Could you check a few things on this model? Use its own coordinates, in mm. Face numbers are marked on the shaded views. A direction names the side the tool comes from. Round coordinates to 2 decimals unless told otherwise and drop trailing zeros. Loops run counter-clockwise (first coordinate to the right, second up) from the corner with the lowest first, then second, coordinate; pieces in that order, holes last. Notation, with made-up numbers: (-9, 28) -> (-4, 28) arc R23 ccw to (-4, 55) -> close; hole circle Ø7 at (61.5, 32.25). An arc over 180 degrees is marked (long way). One line per item, written item: value.
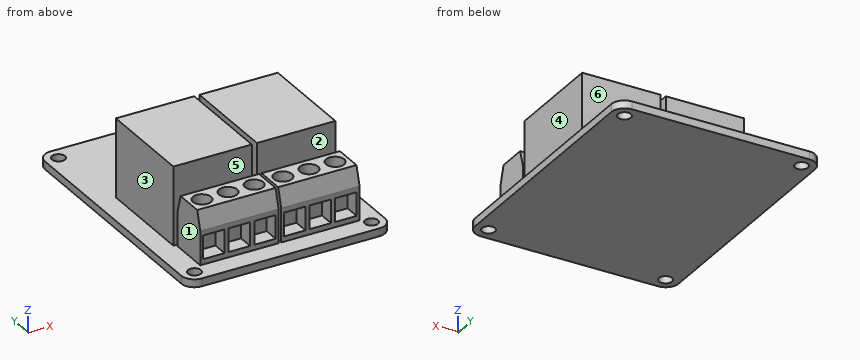
Autodesk Inventor part; units mm, degrees
ref_plane "YZ Plane" through (0, 0, 0) normal (1, 0, 0) x (0, 1, 0)
ref_plane "XZ Plane" through (0, 0, 0) normal (0, 1, 0) x (-1, 0, 0)
ref_plane "XY Plane" through (0, 0, 0) normal (0, 0, 1) x (1, 0, 0)
sketch "Sketch1" plane through (0, 0, 0) normal (0, 0, 1) x (1, 0, 0)
  line L0 (-17, -25) -> (17, -25)
  line L1 (19.5, -22.5) -> (19.5, 22.5)
  line L2 (17, 25) -> (-17, 25)
  line L3 (-19.5, 22.5) -> (-19.5, -22.5)
  line L4 (19.5, -25) -> (-19.5, 25) construction
  circle A0 centre (16.95, -22.45) radius 1.25
  arc A1 (17, -25) -> (19.5, -22.5) centre (17, -22.5) ccw
  circle A2 centre (-16.95, -22.45) radius 1.25
  circle A3 centre (-16.95, 22.45) radius 1.25
  circle A4 centre (16.95, 22.45) radius 1.25
  arc A5 (19.5, 22.5) -> (17, 25) centre (17, 22.5) ccw
  arc A6 (-17, 25) -> (-19.5, 22.5) centre (-17, 22.5) ccw
  arc A7 (-19.5, -22.5) -> (-17, -25) centre (-17, -22.5) ccw
  point P0 (0, 0)
  point P1 (-19.5, -25)
  point P2 (19.5, 25)
  point P3 (0, 0)
  dimension "d0" = 50
  dimension "d1" = 39
  dimension "d2" = 2.5
  dimension "d3" = 2.55
  dimension "d4" = 2.55
  dimension "d5" = 2.5
  dimension "d6" = 2.5
  dimension "d7" = 2.5
  dimension "d8" = 2.5
  dimension "d9" = 2.55
  dimension "d10" = 2.55
  dimension "d11" = 2.55
  dimension "d12" = 2.55
  dimension "d13" = 2.55
  dimension "d14" = 2.55
  dimension "d15" = 2.5
extrude "Extrusion1" add sketch "Sketch1" along normal blind 1.5
sketch "Sketch2" plane through (0, 0, 1.5) normal (0, 0, 1) x (1, 0, 0)
  line L0 (0.5, -13) -> (15.5, -13)
  line L1 (15.5, -13) -> (15.5, 6)
  line L2 (15.5, 6) -> (0.5, 6)
  line L3 (0.5, 6) -> (0.5, -13)
  line L4 (-15.5, -13) -> (-0.5, -13)
  line L5 (-0.5, -13) -> (-0.5, 6)
  line L6 (-0.5, 6) -> (-15.5, 6)
  line L7 (-15.5, 6) -> (-15.5, -13)
  line L8 (19.5, -22.5) -> (19.5, 22.5)
  line L9 (-19.5, 22.5) -> (-19.5, -22.5)
  line L10 (-17, -25) -> (17, -25)
  point P0 (0, 0)
  dimension "d18" = 15
  dimension "d19" = 19
  dimension "d22" = 16
  dimension "d27" = 4
  dimension "d28" = 39
  dimension "d29" = 12
extrude "Extrusion2" add sketch "Sketch2" along normal blind 15
sketch "Sketch3" plane through (0, 0, 1.5) normal (0, 0, 1) x (1, 0, 0)
  line L0 (0, -21) -> (-15, -21)
  line L1 (-15, -21) -> (-15, -13.5)
  line L2 (-15, -13.5) -> (0, -13.5)
  line L3 (0, -13.5) -> (0, -21)
  line L4 (-15.5, -13) -> (-0.5, -13)
  line L5 (-15.5, 6) -> (-15.5, -13)
  line L6 (15.5, -21) -> (0.5, -21)
  line L7 (0.5, -21) -> (0.5, -13.5)
  line L8 (0.5, -13.5) -> (15.5, -13.5)
  line L9 (15.5, -13.5) -> (15.5, -21)
  line L10 (0.5, -13) -> (15.5, -13)
  point P0 (0, 0)
  dimension "d32" = 15
  dimension "d33" = 7.5
  dimension "d34" = 0.5
  dimension "d35" = 0.5
  dimension "d36" = 15
  dimension "d37" = 7.5
  dimension "d38" = 0.5
  dimension "d39" = 0.5
extrude "Extrusion3" add sketch "Sketch3" along normal blind 10
chamfer "Chamfer1" distance 1 distance2 3.5 1 edges at (8, -21, 11.5) measured on face at (10.5, -18.5, 11.5)
chamfer "Chamfer2" distance 1 distance2 3.5 1 edges at (8, -13.5, 11.5) measured on face at (10.5, -17.8333, 11.5)
chamfer "Chamfer3" distance 1 distance2 3.5 1 edges at (-7.5, -13.5, 11.5) measured on face at (-5, -18.5, 11.5)
chamfer "Chamfer4" distance 1 distance2 3.5 1 edges at (-7.5, -21, 11.5) measured on face at (-5, -18.8333, 11.5)
sketch "Sketch4" plane through (0, 0, 11.5) normal (0, 0, 1) x (1, 0, 0)
  line L0 (0.5, -14.5) -> (0.5, -20)
  line L1 (0, -20) -> (0, -14.5)
  line L2 (0.25, -35.642) -> (0.25, -29.5385) construction
  circle A0 centre (-12.5, -17.25) radius 1.75
  line L3 (-15, -14.5) -> (-15, -20)
  line L4 (-15, -14.5) -> (0, -14.5)
  line L5 (0, -20) -> (-15, -20)
  circle A1 centre (-7.5, -17.25) radius 1.75
  circle A2 centre (-2.5, -17.25) radius 1.75
  circle A3 centre (13, -17.25) radius 1.75
  circle A4 centre (8, -17.25) radius 1.75
  circle A5 centre (3, -17.25) radius 1.75
  point P0 (0, 0)
  dimension "d54" = 0.5
  dimension "d55" = 0.25
  dimension "d56" = 3.5
  dimension "d57" = 2.5
  dimension "d58" = 5.5
  dimension "d59" = 2.75
  dimension "d62" = 5
extrude "Extrusion4" cut sketch "Sketch4" against normal blind 3 contours A0 | A1 | A2 | A3 | A4 | A5
sketch "Sketch5" plane through (0.5, -21, 1.5) normal (0, -1, 0) x (1, 0, 0)
  line L0 (0.55, 5.5) -> (4.65, 5.5)
  line L1 (4.65, 5.5) -> (4.65, 1)
  line L2 (4.65, 1) -> (0.55, 1)
  line L3 (0.55, 1) -> (0.55, 5.5)
  line L4 (15, 10) -> (0, 10)
  line L5 (0, 0) -> (0, 6.5)
  line L6 (5.45, 1) -> (5.45, 5.5)
  line L7 (5.45, 5.5) -> (9.55, 5.5)
  line L8 (9.55, 1) -> (5.45, 1)
  line L9 (9.55, 5.5) -> (9.55, 1)
  line L10 (10.35, 1) -> (10.35, 5.5)
  line L11 (10.35, 5.5) -> (14.45, 5.5)
  line L12 (14.45, 1) -> (10.35, 1)
  line L13 (14.45, 5.5) -> (14.45, 1)
  line L14 (15, 0) -> (15, 6.5)
  line L15 (-0.5, 0) -> (-0.5, 6.5)
  line L16 (-0.25, -5.4551) -> (-0.25, -7.5555) construction
  line L17 (-1.05, 5.5) -> (-5.15, 5.5)
  line L18 (-5.15, 5.5) -> (-5.15, 1)
  line L19 (-5.15, 1) -> (-1.05, 1)
  line L20 (-1.05, 1) -> (-1.05, 5.5)
  line L21 (-5.95, 1) -> (-5.95, 5.5)
  line L22 (-5.95, 5.5) -> (-10.05, 5.5)
  line L23 (-10.05, 1) -> (-5.95, 1)
  line L24 (-10.05, 5.5) -> (-10.05, 1)
  line L25 (-10.85, 1) -> (-10.85, 5.5)
  line L26 (-10.85, 5.5) -> (-14.95, 5.5)
  line L27 (-14.95, 1) -> (-10.85, 1)
  line L28 (-14.95, 5.5) -> (-14.95, 1)
  point P0 (-0.5, -1.5)
  dimension "d71" = 4.1
  dimension "d72" = 4.5
  dimension "d73" = 4.5
  dimension "d74" = 0.55
  dimension "d77" = 4.9
  dimension "d85" = 0.5
  dimension "d86" = 0.25
extrude "Extrusion5" cut sketch "Sketch5" against normal blind 3
equation "\"d4\" = d3"
equation "\"d5\" = d2"
equation "\"d6\" = d2"
equation "\"d7\" = d2"
equation "\"d8\" = d2"
equation "\"d9\" = d3"
equation "\"d10\" = d3"
equation "\"d11\" = d3"
equation "\"d12\" = d3"
equation "\"d13\" = d3"
equation "\"d14\" = d3"
equation "\"d15\" = d2"
equation "\"d27\" = -0.5 * d22 + 0.5 * d28 - 0.5 * d18"
equation "\"d39\" = d34"
equation "\"d55\" = 0.5 * d54"
equation "\"d59\" = 0.5 * d58"
equation "\"d86\" = 0.5 * d85"
properties part number "Dual Relay w Breakout Board"
(1) Please list where these lines run through material, in increasing order: L1, parallel to Y at x = 16.95, z = 1.2; L2, parallel to X at y = -6, z = 2.5; L3, parallel to Y at x = 8, z = 10.7.
Results below:
L1: y = -25 to -23.7, -21.2 to 21.2, 23.7 to 25
L2: x = -15.5 to -0.5, 0.5 to 15.5
L3: y = -20.23 to -19, -15.5 to -14.27, -13 to 6
(2) Imagine slicing it at C-C on y = -3. Write out the boundary of the cut face in (x, z).
Results below:
outline: (-19.5, 0) -> (19.5, 0) -> (19.5, 1.5) -> (15.5, 1.5) -> (15.5, 16.5) -> (0.5, 16.5) -> (0.5, 1.5) -> (-0.5, 1.5) -> (-0.5, 16.5) -> (-15.5, 16.5) -> (-15.5, 1.5) -> (-19.5, 1.5) -> close
(3) Imagine slicing it at B-B on x = 3. Write out the boundary of the cut face in (y, z).
Results below:
outline: (-25, 0) -> (25, 0) -> (25, 1.5) -> (6, 1.5) -> (6, 16.5) -> (-13, 16.5) -> (-13, 1.5) -> (-13.5, 1.5) -> (-13.5, 8) -> (-14.5, 11.5) -> (-15.5, 11.5) -> (-15.5, 8.5) -> (-19, 8.5) -> (-19, 11.5) -> (-20, 11.5) -> (-21, 8) -> (-21, 7) -> (-18, 7) -> (-18, 2.5) -> (-21, 2.5) -> (-21, 1.5) -> (-25, 1.5) -> close
(4) Imagine slicing it at D-D on z = 3.75. Give the number of separate pieces and of enclosed holes in the cut face, then the cut area to 3 significant figures.
Results below:
separate pieces: 4
enclosed holes: 0
area: 721 mm²
(5) Imagine slicing it at A-A on z = 12.5. Write out the boundary of the cut face in (x, y), then the cut area to 3 significant figures.
Results below:
outline: (-15.5, -13) -> (-0.5, -13) -> (-0.5, 6) -> (-15.5, 6) -> close; (0.5, -13) -> (15.5, -13) -> (15.5, 6) -> (0.5, 6) -> close
area: 570 mm²
(6) On a 3-axis mill with a long thin cutter (end or side, diameter ignored), from which of +Z, -Z, +X, -X, +Y, -Y can I reach the whole of each face in a straight line? I mean the marked faces 1, 2 and 3. Say none if no direction works.
Results below:
face 1: +Z, -X, -Y
face 2: +Z, +X, -X
face 3: +Z, -X, +Y, -Y
(7) For pin 1 Ø4 at (x, z) = (5.5, 11) entering from -Y; pin 2 Ø2 at (x, z) = (13.5, 5.5) entering from -Y; pin 3 Ø6 at (x, y) = (7, -16.5) entering from +Z; pin 4 Ø1.5 at (x, y) = (2.5, -19) entering from -Z, each with a flat end and sliding along its axis, tell me the tip position at first contact or that it passes through.
Results below:
pin 1: stops at y = -20.71
pin 2: stops at y = -18
pin 3: stops at z = 11.5
pin 4: stops at z = 0
(8) We'd pull the mould along Y, two halves only. Please class the marked faces 4, 5 and 6: +Y half, -Y half, draft (parallel to the pull), parting line (faces both ways), or undercut.
Results below:
face 4: draft
face 5: undercut
face 6: +Y half
